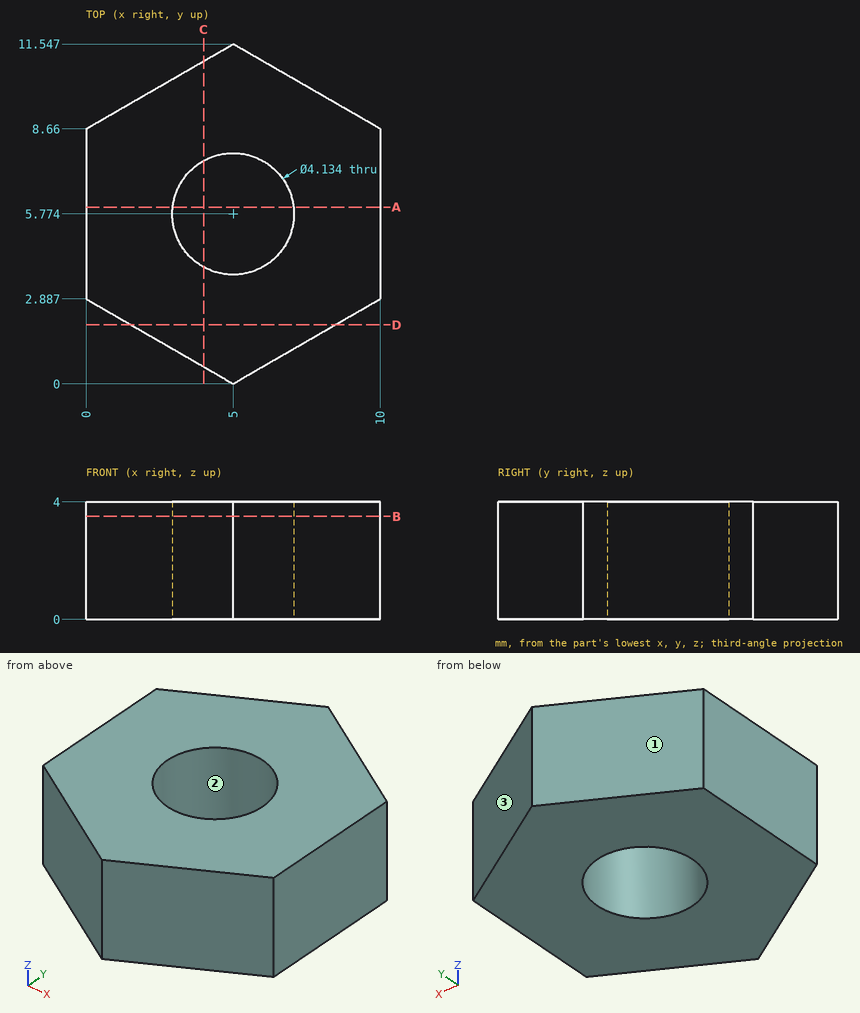
Here's the drawing with two shaded views (mm, measured from the low corner). I have some questions. Give positions to 0.01 mm unless a question says otherwise; leave off trailing zeros. Loops run counter-clockwise (first coordinate to the right, second up) from the corner with the lowest first, then second, coordinate; pieces in that order, holes last. Notation, with made-up numbers: M 66,-1.5 L 110,-1.5 A19 cw 110,3.5 Z; hole C -24,-37.75 d5. An arc over 180 degrees is marked long. One line per item, written item: value. Start each with the question number.
1) Thinking about a two-plate mould opening in X: for the marked faces 1, 2 and 3, which applies, +X half, -X half, draft (parallel to the pull), parting line (faces both ways), or undercut?
2) I'm going to push a flat-ended pin straight in: pin 1 (2.5 mm diameter, centred on x = 5, y = 5.77, fed in from -Z). Where does the tip first touch, or does it pass through?
3) If we section it at C-C, the plane x = 4: Write out the boundary of the cut face in (y, z) (1 decimal).
4) If we section it at A-A, the plane y = 6: Write out the boundary of the cut face in (x, z) (1 decimal).
5) If I drill on line 1 (Y direction, x = 4.25, z = 1.55) (1 decimal); line 2 (Y direction, x = 6.25, z = 1.9) (1 decimal); line 3 (X direction, y = 7, z = 3.7) (1 decimal), over which ranges is the centre line in solid material (lowest first)? Write a range as [from, to].
6) If we section it at D-D, the plane y = 2: Write out the boundary of the cut face in (x, z) (1 decimal).
7) If we section it at B-B, the plane z = 3.5: Write out the boundary of the cut face in (x, y) (1 decimal).
Completed:
1. face 1: -X half
1. face 2: undercut
1. face 3: +X half
2. pin 1: passes through
3. outline: M 0.6,0 L 4,0 L 4,4 L 0.6,4 Z; M 7.6,0 L 11,0 L 11,4 L 7.6,4 Z
4. outline: M 0,0 L 2.9,0 L 2.9,4 L 0,4 Z; M 7.1,0 L 10,0 L 10,4 L 7.1,4 Z
5. line 1: y = [0.4, 3.8], [7.7, 11.1]
5. line 2: y = [0.7, 4.1], [7.4, 10.8]
5. line 3: x = [0, 3.3], [6.7, 10]
6. outline: M 1.5,0 L 8.5,0 L 8.5,4 L 1.5,4 Z
7. outline: M 0,2.9 L 5,0 L 10,2.9 L 10,8.7 L 5,11.5 L 0,8.7 Z; hole C 5,5.8 d4.1
